Autodesk Inventor part; units mm, degrees
ref_plane "YZ Plane" through (0, 0, 0) normal (1, 0, 0) x (0, 1, 0)
ref_plane "XZ Plane" through (0, 0, 0) normal (0, 1, 0) x (-1, 0, 0)
ref_plane "XY Plane" through (0, 0, 0) normal (0, 0, 1) x (1, 0, 0)
sketch "Base" plane through (0, 0, 0) normal (0, 0, 1) x (1, 0, 0)
  line L0 (0, 0) -> (-24.7487, 24.7487)
  line L1 (0, 0) -> (35, 0) construction
  line L2 (-24.7487, 24.7487) -> (-24.7487, 0)
  line L3 (-24.7487, 0) -> (0, 0)
  line L4 (-24.7487, 24.7487) -> (-27.7487, 24.7487)
  line L5 (-27.7487, 24.7487) -> (-27.7487, 0)
  line L6 (-27.7487, 0) -> (-24.7487, 0)
  line L7 (-24.7487, 0) -> (-24.7487, 24.7487)
  line L8 (-27.7487, 0) -> (17.2513, 0)
  line L9 (17.2513, 0) -> (17.2513, -5)
  line L10 (17.2513, -5) -> (-27.7487, -5)
  line L11 (-27.7487, -5) -> (-27.7487, 0)
  line L12 (3, 15.0208) -> (-9.7279, 27.7487)
  line L13 (-9.7279, 27.7487) -> (-27.7487, 9.7279)
  line L14 (-27.7487, 9.7279) -> (-15.0208, -3)
  line L15 (-15.0208, -3) -> (3, 15.0208)
  line L16 (3, 15.0208) -> (-27.7487, 9.7279) construction
  line L17 (-9.7279, 27.7487) -> (-15.0208, -3) construction
  line L18 (-24.9203, 9.7279) -> (-9.7279, 24.9203)
  line L19 (-9.7279, 24.9203) -> (0.1716, 15.0208)
  line L20 (0.1716, 15.0208) -> (-15.0208, -0.1716)
  line L21 (-15.0208, -0.1716) -> (-24.9203, 9.7279)
  line L22 (-18.7383, 18.7383) -> (-17.3241, 17.3241)
  line L23 (-7.4246, 7.4246) -> (-6.0104, 6.0104)
  line L24 (-27.7487, 9.7279) -> (-23.5061, 13.9706)
  line L25 (-23.5061, 13.9706) -> (-22.0919, 12.5564)
  line L26 (-22.0919, 12.5564) -> (-26.3345, 8.3137)
  line L27 (-26.3345, 8.3137) -> (-27.7487, 9.7279)
  line L28 (-23.5061, 5.4853) -> (-19.2635, 1.2426)
  line L29 (-16.435, 4.0711) -> (-23.5061, 5.4853) construction
  line L30 (-20.6777, 8.3137) -> (-19.2635, 1.2426) construction
  line L31 (-6.0104, 6.0104) -> (-7.4246, 7.4246)
  line L32 (-7.4246, 7.4246) -> (-16.435, -1.5858)
  line L33 (-16.435, -1.5858) -> (-15.0208, -3)
  line L34 (-15.0208, -3) -> (-6.0104, 6.0104)
  line L35 (-15.0208, -0.1716) -> (-17.8492, 2.6569)
  line L36 (-17.8492, 2.6569) -> (-19.2635, 1.2426)
  line L37 (-19.2635, 1.2426) -> (-16.435, -1.5858)
  line L38 (-16.435, -1.5858) -> (-15.0208, -0.1716)
  line L39 (-26.3345, 8.3137) -> (-23.5061, 5.4853)
  line L40 (-23.5061, 5.4853) -> (-22.0919, 6.8995)
  line L41 (-22.0919, 6.8995) -> (-24.9203, 9.7279)
  line L42 (-24.9203, 9.7279) -> (-26.3345, 8.3137)
  point P0 (-12.3744, 12.3744)
  point P1 (-19.9706, 4.7782)
  dimension "d0" = 35
  dimension "d1" = 135
  dimension "d2" = 3
  dimension "d3" = 45
  dimension "d4" = 5
  dimension "d5" = 18
  dimension "d6" = 2
  dimension "d7" = 6
extrude "Extrusion1" add sketch "Base" along normal blind 5.5 contours L3 L15 L0 | L8 L9 L10 L11 L6 L3 L14 L15 | L15 L3 L20 L0 | L15 L14 L32 L20 L3 | L20 L3 L21 L2 L18 L0 | L20 L21 L3 | L18 L25 L13 L0 | L21 L32 L14 L3 | L3 L14 L36 L21 | L13 L2 L0 | L18 L2 L13 L25 | L3 L2 L14 | L36 L14 L40 L21 | L5 L14 L2 L6 | L2 L13 L5 L4 | L18 L26 L14 L13 L2 | L2 L21 L18 | L40 L14 L2 L21 | L2 L14 L26 L21
extrude "Extrusion2" add sketch "Base" along normal blind 12.5 contours L15 L3 L20 L0 | L15 L14 L32 L20 L3 | L21 L32 L14 L3 | L3 L14 L36 L21 | L18 L2 L13 L25 | L18 L26 L14 L13 L2 | L40 L14 L2 L21 | L2 L14 L26 L21
sketch "TouchProtection" plane through (0, 0, 12.5) normal (0, 0, 1) x (1, 0, 0)
  line L0 (-6.0104, 6.0104) -> (-15.0208, -3)
  line L1 (-6.0104, 6.0104) -> (-15.0208, -3)
  line L2 (-15.0208, -3) -> (-27.6905, 9.6697)
  line L3 (-27.6905, 9.6697) -> (-18.6801, 18.6801)
  line L4 (-18.6801, 18.6801) -> (-6.0104, 6.0104)
  point P0 (0, 0)
extrude "Extrusion3" add sketch "TouchProtection" along normal blind 2
sketch "MountingHolesBottom" plane through (-27.7487, -5, 0) normal (0, -1, 0) x (1, 0, 0)
  line L0 (0, 0) -> (5, 0)
  line L1 (45, 0) -> (40, 0)
  circle A0 centre (5, 0) radius 1.75
  circle A1 centre (40, 0) radius 1.75
  line L2 (5, 0) -> (5, 3)
  line L3 (5, 0) -> (8, 0) construction
  line L4 (6.7321, 3) -> (8.4641, 0)
  line L5 (8.4641, 0) -> (6.7321, -3)
  line L6 (6.7321, -3) -> (3.2679, -3)
  line L7 (3.2679, -3) -> (1.5359, 0)
  line L8 (1.5359, 0) -> (3.2679, 3)
  line L9 (3.2679, 3) -> (6.7321, 3)
  line L10 (40, 0) -> (40, 3)
  line L11 (41.7321, 3) -> (43.4641, 0)
  line L12 (43.4641, 0) -> (41.7321, -3)
  line L13 (41.7321, -3) -> (38.2679, -3)
  line L14 (38.2679, -3) -> (36.5359, 0)
  line L15 (36.5359, 0) -> (38.2679, 3)
  line L16 (38.2679, 3) -> (41.7321, 3)
  line L17 (1.5359, 0) -> (43.4641, 0)
  point P0 (27.7487, 0)
  dimension "d15" = 5
  dimension "d16" = 5
  dimension "d17" = 3.5
  dimension "d18" = 3.5
  dimension "d19" = 3
  dimension "d20" = 90
  dimension "d21" = 3
extrude "Extrusion4" cut sketch "MountingHolesBottom" against normal blind 10 contours A0 L2 L0 | L0 L17 A0 | L2 A0 L17 | L17 L1 A1 | A1 L10 L17 | A1 L1 L10
extrude "Extrusion5" cut sketch "MountingHolesBottom" against normal blind 6 contours L8 L9 L2 A0 L0 | L0 A0 L17 L5 L6 L7 | L15 L16 L10 A1 L17 | L17 A1 L1 L12 L13 L14 | L2 L9 L4 L17 A0 | L16 L11 L1 A1 L10
extrude "Extrusion6" add sketch "MountingHolesBottom" against normal blind 2.5 contours L8 L9 L2 A0 L0 | L0 A0 L17 L5 L6 L7 | L15 L16 L10 A1 L17 | L17 A1 L1 L12 L13 L14 | L2 L9 L4 L17 A0 | L16 L11 L1 A1 L10
sketch "MountingHolesE27" plane through (0, 0, 0) normal (0.7071, 0.7071, 0) x (-0.7071, 0.7071, 0)
  line L0 (0, 0) -> (0, 5.5)
  line L1 (0, 0) -> (8.5, 0)
  line L2 (0, 0) -> (35, 0)
  line L3 (8.5, 0) -> (26.5, 0)
  circle A0 centre (8.5, 0) radius 1.75
  circle A1 centre (26.5, 0) radius 1.75
  line L4 (8.5, 0) -> (8.5, 3)
  line L5 (26.5, 0) -> (26.5, 3)
  line L6 (26.5, 0) -> (29.5, 0) construction
  line L7 (28.2321, 3) -> (29.9641, 0)
  line L8 (29.9641, 0) -> (28.2321, -3)
  line L9 (28.2321, -3) -> (24.7679, -3)
  line L10 (24.7679, -3) -> (23.0359, 0)
  line L11 (23.0359, 0) -> (24.7679, 3)
  line L12 (24.7679, 3) -> (28.2321, 3)
  line L13 (10.2321, 3) -> (11.9641, 0)
  line L14 (11.9641, 0) -> (10.2321, -3)
  line L15 (10.2321, -3) -> (6.7679, -3)
  line L16 (6.7679, -3) -> (5.0359, 0)
  line L17 (5.0359, 0) -> (6.7679, 3)
  line L18 (6.7679, 3) -> (10.2321, 3)
  dimension "d30" = 8.5
  dimension "d31" = 18
  dimension "d32" = 180
  dimension "d33" = 3.5
  dimension "d34" = 3.5
  dimension "d35" = 3
  dimension "d36" = 3
  dimension "d37" = 90
extrude "Extrusion8" cut sketch "MountingHolesE27" against normal blind 10 contours A0 L4 L1 | L1 L2 A0 | L4 A0 L2 | A1 L5 L2 | L2 A1 | L5 A1 L2
extrude "Extrusion9" cut sketch "MountingHolesE27" against normal blind 7 contours L17 L18 L4 A0 L1 | L1 A0 L2 L14 L15 L16 | L11 L12 L5 A1 L2 | L2 A1 L8 L9 L10 | L4 L18 L13 L2 A0 | L5 L12 L7 L2 A1
extrude "Extrusion10" add sketch "MountingHolesE27" against normal blind 4 contours L17 L18 L4 A0 L1 | L1 A0 L2 L14 L15 L16 | L11 L12 L5 A1 L2 | L2 A1 L8 L9 L10 | L4 L18 L13 L2 A0 | L5 L12 L7 L2 A1
sketch "Sketch7" plane through (0, 0, 0) normal (0, 0, -1) x (-1, 0, 0)
  line L0 (-17.2513, -5) -> (-17.2513, 0)
  line L1 (24.7487, 24.7487) -> (27.7487, 24.7487)
  line L2 (-17.2513, -5) -> (27.7487, -5)
  line L3 (27.7487, -5) -> (27.7487, 24.7487)
  line L4 (27.7487, 24.7487) -> (-17.2513, 24.7487)
  line L5 (-17.2513, 24.7487) -> (-17.2513, -5)
  point P0 (0, 0)
extrude "Extrusion11" cut sketch "Sketch7" along normal blind 21.25
sketch "Sketch8" plane through (0, 0, 0) normal (0, 0, -1) x (-1, 0, 0)
  line L0 (7.2478, 7.2478) -> (17.5009, 17.5009)
  line L1 (12.3744, 12.3744) -> (13.0815, 11.6673)
  line L2 (12.3744, 12.3744) -> (13.3744, 12.3744) construction
  line L3 (13.0815, 11.6673) -> (15.9099, 8.8388)
  line L4 (18.4555, 5.7276) -> (12.7986, 11.3844)
  line L5 (12.7986, 11.3844) -> (13.3643, 11.9501)
  line L6 (13.3643, 11.9501) -> (19.0212, 6.2933)
  line L7 (19.0212, 6.2933) -> (18.4555, 5.7276)
  line L8 (18.4555, 5.7276) -> (13.3643, 11.9501) construction
  line L9 (12.7986, 11.3844) -> (19.0212, 6.2933) construction
  line L10 (-10.5258, -5.0105) -> (-2.5258, -5.0105)
  line L11 (20.9987, -5) -> (-10.5013, -5)
  line L12 (-10.5258, -5.0105) -> (-2.5258, -5.0105) construction
  line L13 (-2.5258, -5.0105) -> (-2.5258, -2.5105)
  line L14 (-6.5258, -2.1105) -> (1.4742, -2.1105)
  line L15 (1.4742, -2.1105) -> (1.4742, -2.9105)
  line L16 (1.4742, -2.9105) -> (-6.5258, -2.9105)
  line L17 (-6.5258, -2.9105) -> (-6.5258, -2.1105)
  line L18 (-6.5258, -2.1105) -> (1.4742, -2.9105) construction
  line L19 (1.4742, -2.1105) -> (-6.5258, -2.9105) construction
  point P0 (0, 0)
  dimension "d46" = 1
  dimension "d47" = 45
  dimension "d48" = 4
  dimension "d49" = 0.8
  dimension "d50" = 8
  dimension "d51" = 0
  dimension "d52" = 2.5
  dimension "d53" = 8
  dimension "d54" = 0.8
extrude "Extrusion12" cut sketch "Sketch8" against normal blind 4
properties part number "e27_Holder_v2"
Verification items for the finished model (mm, model axes). A direction names the side the tool comes from. Give positions to 0.01 mm unless a question says otherwise; leave off trailing zeros. Loops run counter-clockwise (first coordinate to the right, second up) from the corner with the lowest first, then second, coordinate; pieces in that order, holes last. Notation, with made-up numbers: M 13,9 L 71,9 A15 ccw 71,22 Z; hole C 31,23 d10. An arc over 180 degrees is marked long. Return JSON: item names as keys, results as strings.
1) Gauge pin test, flat ends, axial feed: P1, Ø1.4, axis at x = -22.5, z = 0.5, coming from the -Y side; P2, Ø1.7, axis at x = 11, z = 4, coming from the +Y side; P3, Ø1.7, axis at x = -22, y = 0, coming from the -Z side. Record the tip position at first contact, or that the pin passes through.
Findings:
{"P1": "stops at y = 5", "P2": "stops at y = 0", "P3": "stops at z = 3"}
2) Section check A-A, the plane z = 7.75. Enter the section's corners in (x, y).
Findings:
{"outline": "M -27.75,9.73 L -23.51,5.49 L -22.09,6.9 L -24.92,9.73 L -22.09,12.56 L -23.51,13.97 Z; M -19.26,1.24 L -15.02,-3 L -6.01,6.01 L -7.42,7.42 L -15.02,-0.17 L -17.85,2.66 Z"}
3) Mould release check, pull along Z, two halves, no side actions. Record for faces 1 (the flat face through (16, -3, 0)), 2 (the flat face through (-26, 24.749, 3)), 3 (the flat face through (-16, 7, 5.5)), 4 (the flat face through (-23.53, 11.12, 8.95)): released by +Z, released by -Z, zero draft, split by the parting line, or undercut.
Findings:
{"face 1": "released by -Z", "face 2": "zero draft", "face 3": "undercut", "face 4": "undercut"}
4) Material ranges on L1, parallel to Z at x = -13.5, y = 12.75; L2, parallel to Y at x = 5.5, z = 2.5; L3, parallel to Z at x = 8.5, y = -3.5, recorded low to high. Write a range as [from, to].
Findings:
{"L1": "z = [0, 5.5], [12.5, 14.5]", "L2": "y = [-5, -2.91], [-2.11, 0]", "L3": "z = [0, 5.5]"}
5) Section check C-C, the plane x = 14.5. Enter the section's corners in (y, z).
Findings:
{"outline": "M -5,0 L -2.5,0 L -2.5,2.11 L 0,2.11 L 0,5.5 L -5,5.5 Z"}
6) Section check B-B, the plane z = 2.5. Count the separate pieces of the cut face and the enclosed holes in it, and give its area (3 significant figures).
Findings:
{"separate pieces": "1", "enclosed holes": "5", "area": "544 mm2"}
7) Section check D-D, the plane y = 8. Enter the section's corners in (x, z), and give its area (3 significant figures).
Findings:
{"outline": "M -27.75,0 L -17.31,0 L -17.31,4 L -16.18,4 L -16.18,0 L -8,0 L -8,5.5 L -23.19,5.5 L -23.19,12.5 L -8,12.5 L -8,14.5 L -26.02,14.5 L -26.02,5.5 L -27.75,5.5 Z", "area": "160 mm2"}
8) Tool access check on faces 5 (the flat face through (-22.81, 6.18, 8.95)), 6 (the flat face through (-21.296, 3.275, 12.937)), 7 (the flat face through (-18.546, 1.96, 8.951)). Record the directions out of +Z, -Z, +X, -X, +Y, -Y that give a thin tool (end or side, any length) a straight path to the whole face; none if there is none.
Findings:
{"face 5": "-Y", "face 6": "+Z, -X, -Y", "face 7": "-X, +Y"}
